Drawing for the job (mm, zero at the part's lowest x, y, z). Coordinates: 2 decimals unless noted, no trailing zeros. Write each loop counter-clockwise with the first axis right and the second up, starting at its lowest first coordinate (ties: lowest second). Pieces come first, ordered by that corner, then holes. Notation, with made-up numbers: (13, 31) - (70, 31) arc R7 ccw to (70, 40) - close; hole circle Ø7 at (17, -3). An arc over 180 degrees is marked (long way). Write each question's results on one line, items separated by ' | '.
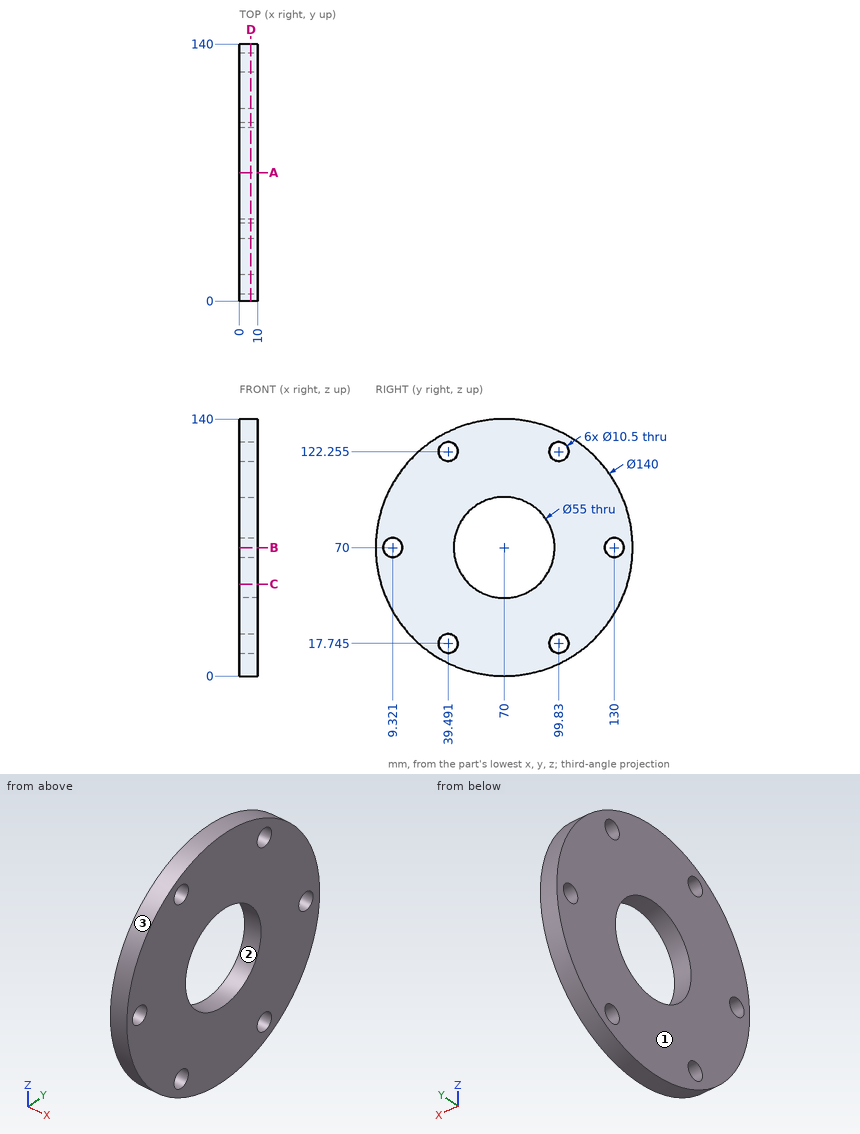
(1) Saw through at D-D on x = 6.25. Count the separate pieces of the cut face and the enclosed holes in it, then the cut area to 3 significant figures.
Return value:
separate pieces: 1 | enclosed holes: 7 | area: 12,500 mm^2
(2) Wall check: line 1 (Z direction, x = 8, y = 64); line 2 (Y direction, x = 9, z = 118.5) (1 decimal); line 3 (Y direction, x = 9.5, z = 69) (1 decimal). Give the ranges that are in metal, low to high. Write a range as from..to.
Return value:
line 1: z = 0.26..43.16, 96.84..139.74 | line 2: y = 19.5..35.8, 43.2..96.2, 103.5..120.5 | line 3: y = 0..4.2, 14.5..42.5, 97.5..124.8, 135.2..140
(3) Saw through at B-B on z = 70. Write the cut outline in (x, y), then the cut area to 3 significant figures.
Return value:
outline: (0, 0) - (10, 0) - (10, 4.07) - (0, 4.07) - close; (0, 14.57) - (10, 14.57) - (10, 42.5) - (0, 42.5) - close; (0, 97.5) - (10, 97.5) - (10, 124.75) - (0, 124.75) - close; (0, 135.25) - (10, 135.25) - (10, 140) - (0, 140) - close | area: 640 mm^2
(4) Two-plate mould, pull along Z, no slides. Class the marked faces 1, 2 and 3: released by +Z, released by -Z, zero draft, split by the parting line, or undercut.
Return value:
face 1: zero draft | face 2: undercut | face 3: split by the parting line
(5) Flat gauge pins, fed straight in: P1, Ø4, axis at x = 2.5, y = 89, coming from the +Z side (1 decimal); P2, Ø12, axis at y = 9.32, z = 70, coming from the +X side; P3, Ø6, axis at x = 8.5, z = 17.5, coming from the -Y side (1 decimal); P4, Ø4, axis at x = 5, y = 125.5, coming from the -Z side. Where does each tip first touch, or does it go through?
Return value:
P1: stops at z = 137.9 | P2: stops at x = 10 | P3: stops at y = 20.5 | P4: stops at z = 24.86
(6) Saw through at C-C on z = 50. Write the cut outline in (x, y) (1 decimal).
Return value:
outline: (0, 2.9) - (10, 2.9) - (10, 51.1) - (0, 51.1) - close; (0, 88.9) - (10, 88.9) - (10, 137.1) - (0, 137.1) - close
(7) Saw through at A-A on y = 70. Write the cut outline in (x, z).
Return value:
outline: (0, 0) - (10, 0) - (10, 42.5) - (0, 42.5) - close; (0, 97.5) - (10, 97.5) - (10, 140) - (0, 140) - close
